The model under review builds one solid part; all positions refer to its coordinate system, in mm. Face numbers are marked on the shaded views. A direction names the side the tool comes from. Give positions to 0.01 mm unless a question says otherwise; leave off trailing zeros. Order: outer loops, then holes, each group sorted by start corner. A loop starts at its lowest first (then second) coordinate and runs counter-clockwise, first axis right, second up. Notation, with made-up numbers: (-35, 21) -> (-23, 21) arc R8 cw to (-23, 32) -> close; hole circle Ø6 at (79.25, 8.25). An arc over 180 degrees is marked (long way). Use one line per item in the form item = value.
Autodesk Inventor part; units mm, degrees
ref_plane "YZ Plane" through (0, 0, 0) normal (1, 0, 0) x (0, 1, 0)
ref_plane "XZ Plane" through (0, 0, 0) normal (0, 1, 0) x (-1, 0, 0)
ref_plane "XY Plane" through (0, 0, 0) normal (0, 0, 1) x (1, 0, 0)
sketch "Sketch1" plane through (0, 0, 0) normal (0, 1, 0) x (-1, 0, 0)
  circle A0 centre (0, 0) radius 1.5
  circle A1 centre (0, 0) radius 2.5
  dimension "d0" = 3
  dimension "d1" = 5
extrude "Extrusion1" add sketch "Sketch1" along normal blind 10 contours A0
extrude "Extrusion2" add sketch "Sketch1" against normal blind 2 contours A0 | A1
fillet "Fillet1" radius 0.5 1 edges at (2.5, -2, 0)
sketch "Sketch2" plane through (0, -2, 0) normal (0, -1, 0) x (1, 0, 0)
  circle A0 centre (0, 0) radius 1.5
  line L0 (0, 0.5) -> (1.4142, 0.5)
  line L1 (1.4142, 0.5) -> (1.4142, -0.5)
  line L2 (1.4142, -0.5) -> (0, -0.5)
  line L3 (0, -0.5) -> (0, 0.5)
  dimension "d7" = 1
  dimension "d8" = 0.5
extrude "Extrusion3" cut sketch "Sketch2" against normal blind 2 contours L1 L2 L3 L0
pattern_circular "Circular Pattern1" count 4 over 360 about axis through (0, 0, 0) along (0, -1, 0) of "Extrusion3"
thread "Thread1"
chamfer "Chamfer1" distance 1 angle 45 1 edges at (1.5, 10, 0)
properties part number "KisLemezcsavar"
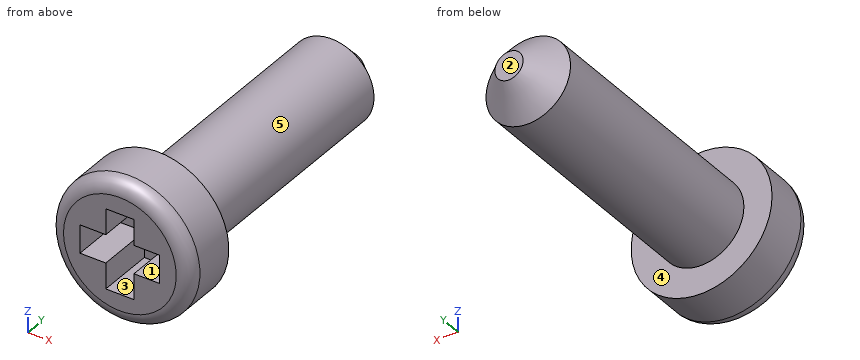
1. For pin 1 Ø1 at (x, y) = (-1, -0.5) entering from +Z; pin 2 Ø1 at (y, z) = (-1.5, -1) entering from +X; pin 3 Ø0.7 at (y, z) = (-1.5, 1) entering from -X, all flat-tipped, find the tip position at first contact; note any pin that passes through.
Values:
pin_1 = 2.45
pin_2 = 2.45
pin_3 = -2.41
2. Add section C-C on y = 1.5. Give the boundary of the cut face in (x, z), then the cut area to 3 significant figures.
Values:
outline = circle Ø3 at (0, 0)
area = 7.07 mm^2
3. Add section A-A on x = 0. Give the boundary of the cut face in (y, z), then the cut area to 3 significant figures.
Values:
outline = (-2, -2) arc R0.5 ccw to (-1.5, -2.5) -> (0, -2.5) -> (0, -1.5) -> (9, -1.5) -> (10, -0.5) -> (10, 0.5) -> (9, 1.5) -> (0, 1.5) -> (0, 2.5) -> (-1.5, 2.5) arc R0.5 ccw to (-2, 2) -> (-2, 1.41) -> (0, 1.41) -> (0, -1.41) -> (-2, -1.41) -> close
area = 33.2 mm^2
4. Add section B-B on z = 0. Give the boundary of the cut face in (x, y).
Values:
outline = (-2.5, -1.5) arc R0.5 ccw to (-2, -2) -> (-1.41, -2) -> (-1.41, 0) -> (1.41, 0) -> (1.41, -2) -> (2, -2) arc R0.5 ccw to (2.5, -1.5) -> (2.5, 0) -> (1.5, 0) -> (1.5, 9) -> (0.5, 10) -> (-0.5, 10) -> (-1.5, 9) -> (-1.5, 0) -> (-2.5, 0) -> close
5. Tool access review of the marked faces 1 and 2: name each direction out of +Z, -Z, +X, -X, +Y, -Y from which nothing blocks a thin tool from reaching the whole face with its end or side.
Values:
face_1 = -Y
face_2 = +Z, -Z, +X, -X, +Y
6. The part is to be moulded in two halves that separate along Z. For the marked faces 3, 4 and 5, say which applies: +Z half, -Z half, draft (parallel to the pull), parting line (faces both ways), or undercut.
Values:
face_3 = undercut
face_4 = draft
face_5 = parting line
7. For L1, parallel to Y at x = 0.85, z = -1.4; L2, parallel to X at y = 1.5, z = -0.5, list the stretches that pass through material, from the lowest coordinate up.
Values:
L1 = -2 to 0
L2 = -1.41 to 1.41
